Build history of the part. All positions in model axes, mm. A direction names the side the tool comes from. Coordinates: 2 decimals unless noted, no trailing zeros.
```python
from build123d import *

# Parameters (mm, degrees)
SKETCH_W        = 150
SKETCH_H        = 115
PAD_DEPTH       = 3
SKETCH001_W     = 150
SKETCH001_H     = 3
PAD001_DEPTH    = 40
SKETCH002_R     = 3.5
SKETCH002_R_2   = 1.5
PAD002_DEPTH    = 7
SKETCH003_R     = 8.2
SKETCH003_R_2   = 2.25
POCKET_DEPTH    = 5
SKETCH004_R     = 3.65
SKETCH004_R_2   = 1.6
POCKET001_DEPTH = 5
PAD003_DEPTH    = 9
POCKET002_DEPTH = 8
SKETCH007_R     = 2.956815
SKETCH007_R_2   = 3.91912
POCKET003_DEPTH = 5
SKETCH008_R     = 3.375
POCKET004_DEPTH = 5
POCKET005_DEPTH = 5
SKETCH012_W     = 6
SKETCH012_H     = 8
PAD006_DEPTH    = 8
SKETCH013_W     = 6
SKETCH013_H     = 8
PAD007_DEPTH    = 8
SKETCH016_R     = 1.5
POCKET008_DEPTH = 10
SKETCH017_R     = 1.5
POCKET009_DEPTH = 10
FILLET001_R     = 2
FILLET002_R     = 1.5


with BuildPart() as part:
    # Sketch → Pad (new body)
    with BuildSketch(Plane.XY):
        with Locations((99.883204, -84.177484)):
            Rectangle(SKETCH_W, SKETCH_H)
    extrude(amount=PAD_DEPTH)

    # Sketch001 (on Face6 of Pad) → Pad001 (join)
    with BuildSketch(Plane.XY.offset(3)):
        with Locations((99.883211, -140.17749)):
            Rectangle(SKETCH001_W, SKETCH001_H)
        with Locations((99.883211, -28.1775)):
            Rectangle(SKETCH001_W, SKETCH001_H)
    extrude(amount=PAD001_DEPTH)

    # Sketch002 (on Face5 of Pad001) → Pad002 (join)
    with BuildSketch(Plane.XY.offset(3)):
        with Locations((45.316391, -43.665684)):
            Circle(SKETCH002_R)
        with Locations((45.316391, -43.665684)):
            Circle(SKETCH002_R_2, mode=Mode.SUBTRACT)
        with Locations((134.578049, -43.803013)):
            Circle(SKETCH002_R)
        with Locations((134.578049, -43.803013)):
            Circle(SKETCH002_R_2, mode=Mode.SUBTRACT)
        with Locations((45.316391, -133.064651)):
            Circle(SKETCH002_R)
        with Locations((45.316391, -133.064651)):
            Circle(SKETCH002_R_2, mode=Mode.SUBTRACT)
        with Locations((134.578049, -132.927338)):
            Circle(SKETCH002_R)
        with Locations((134.578049, -132.927338)):
            Circle(SKETCH002_R_2, mode=Mode.SUBTRACT)
    extrude(amount=PAD002_DEPTH)

    # Sketch003 (on Face8 of Pad002) → Pocket (cut)
    with BuildSketch(Plane(origin=(0, -26.6775, 0), x_dir=(-1, 0, 0), z_dir=(0, 1, 0))):
        with Locations((-155.160995, 22.957462)):
            Circle(SKETCH003_R)
        with Locations((-128.150894, 23.01816)):
            Circle(SKETCH003_R)
        with Locations((-164.297668, 32.157272)):
            Circle(SKETCH003_R_2)
        with Locations((-145.858627, 32.062714)):
            Circle(SKETCH003_R_2)
        with Locations((-164.113113, 13.90062)):
            Circle(SKETCH003_R_2)
        with Locations((-145.905151, 13.821107)):
            Circle(SKETCH003_R_2)
        with Locations((-137.079453, 32.188087)):
            Circle(SKETCH003_R_2)
        with Locations((-137.091354, 13.88285)):
            Circle(SKETCH003_R_2)
        with Locations((-118.778183, 32.004562)):
            Circle(SKETCH003_R_2)
        with Locations((-118.969612, 14.010464)):
            Circle(SKETCH003_R_2)
        with Locations((-109.972557, 13.819037)):
            Circle(SKETCH003_R_2)
        with Locations((-109.969048, 32.209045)):
            Circle(SKETCH003_R_2)
        with Locations((-91.723251, 32.195992)):
            Circle(SKETCH003_R_2)
        with Locations((-91.787064, 13.88285)):
            Circle(SKETCH003_R_2)
        with Locations((-101.261856, 22.888664)):
            Circle(SKETCH003_R)
    extrude(amount=-POCKET_DEPTH, mode=Mode.SUBTRACT)

    # Sketch004 (on Face19 of Pocket) → Pocket001 (cut)
    with BuildSketch(Plane.XZ.offset(141.67749)):
        with Locations((87.170862, 25.966157)):
            Circle(SKETCH004_R)
        with Locations((124.674583, 25.581327)):
            Circle(SKETCH004_R)
        with Locations((61.41629, 22.568558)):
            Circle(SKETCH004_R_2)
        with Locations((54.032642, 22.454962)):
            Circle(SKETCH004_R_2)
    extrude(amount=-POCKET001_DEPTH, mode=Mode.SUBTRACT)

    # Sketch005 (on Face8 of Pocket001) → Pad003 (join)
    with BuildSketch(Plane(origin=(0, -26.6775, 0), x_dir=(-1, 0, 0), z_dir=(0, 1, 0))):
        with BuildLine():
            ThreePointArc((-71.425017, 25.728505), (-79.425017, 17.728505), (-71.425017, 9.728505))
            Line((-71.425017, 9.728505), (-56.425017, 9.728505))
            ThreePointArc((-56.425017, 9.728505), (-48.425017, 17.728505), (-56.425017, 25.728505))
            Line((-71.425017, 25.728505), (-56.425017, 25.728505))
        make_face()
    extrude(amount=-PAD003_DEPTH)

    # Sketch006 (on Face58 of Pad003) → Pocket002 (cut)
    with BuildSketch(Plane(origin=(0, -26.6775, 0), x_dir=(-1, 0, 0), z_dir=(0, 1, 0))):
        with BuildLine():
            ThreePointArc((-71.144104, 24.608639), (-78.144104, 17.608639), (-71.144104, 10.608639))
            Line((-71.144104, 10.608639), (-56.644104, 10.608639))
            ThreePointArc((-56.644104, 10.608639), (-49.644104, 17.608639), (-56.644104, 24.608639))
            Line((-71.144104, 24.608639), (-56.644104, 24.608639))
        make_face()
    extrude(amount=-POCKET002_DEPTH, mode=Mode.SUBTRACT)

    # Sketch007 (on Face54 of Pocket002) → Pocket003 (cut)
    with BuildSketch(Plane(origin=(0, -34.6775, 0), x_dir=(-1, 0, 0), z_dir=(0, 1, 0))):
        with Locations((-71.614014, 15.088903)):
            Circle(SKETCH007_R)
        with Locations((-56.978443, 19.166483)):
            Circle(SKETCH007_R_2)
    extrude(amount=-POCKET003_DEPTH, mode=Mode.SUBTRACT)

    # Sketch008 (on Face19 of Pocket003) → Pocket004 (cut)
    with BuildSketch(Plane.XZ.offset(141.67749)):
        with Locations((161.787576, 25.778181)):
            Circle(SKETCH008_R)
        with Locations((35.800133, 25.778181)):
            Circle(SKETCH008_R)
        with Locations((105.628538, 25.778181)):
            Circle(SKETCH008_R)
        with Locations((145.6931, 25.778181)):
            Circle(SKETCH008_R)
    extrude(amount=-POCKET004_DEPTH, mode=Mode.SUBTRACT)

    # Sketch009 (on Face5 of Pocket004) → Pocket005 (cut)
    with BuildSketch(Plane.XY.offset(3)):
        with BuildLine():
            ThreePointArc((39.81937, -90.12404), (42.31937, -92.62404), (44.81937, -90.12404))
            Line((44.81937, -90.12404), (44.81937, -60.12404))
            ThreePointArc((44.81937, -60.12404), (42.31937, -57.62404), (39.81937, -60.12404))
            Line((39.81937, -90.12404), (39.81937, -60.12404))
        make_face()
        with BuildLine():
            ThreePointArc((47.81937, -90.124041), (50.31937, -92.624041), (52.81937, -90.124041))
            Line((52.81937, -90.124041), (52.81937, -60.124041))
            ThreePointArc((52.81937, -60.124041), (50.31937, -57.624041), (47.81937, -60.124041))
            Line((47.81937, -90.124041), (47.81937, -60.124041))
        make_face()
        with BuildLine():
            ThreePointArc((55.81937, -90.12404), (58.31937, -92.62404), (60.81937, -90.12404))
            Line((60.81937, -90.12404), (60.81937, -60.12404))
            ThreePointArc((60.81937, -60.12404), (58.31937, -57.62404), (55.81937, -60.12404))
            Line((55.81937, -90.12404), (55.81937, -60.12404))
        make_face()
        with BuildLine():
            ThreePointArc((63.81937, -90.124041), (66.31937, -92.624041), (68.81937, -90.124041))
            Line((68.81937, -90.124041), (68.81937, -60.124041))
            ThreePointArc((68.81937, -60.124041), (66.31937, -57.624041), (63.81937, -60.124041))
            Line((63.81937, -90.124041), (63.81937, -60.124041))
        make_face()
        with BuildLine():
            ThreePointArc((71.81937, -90.12404), (74.31937, -92.62404), (76.81937, -90.12404))
            Line((76.81937, -90.12404), (76.81937, -60.12404))
            ThreePointArc((76.81937, -60.12404), (74.31937, -57.62404), (71.81937, -60.12404))
            Line((71.81937, -90.12404), (71.81937, -60.12404))
        make_face()
        with BuildLine():
            ThreePointArc((79.81937, -90.12404), (82.31937, -92.62404), (84.81937, -90.12404))
            Line((84.81937, -90.12404), (84.81937, -60.12404))
            ThreePointArc((84.81937, -60.12404), (82.31937, -57.62404), (79.81937, -60.12404))
            Line((79.81937, -90.12404), (79.81937, -60.12404))
        make_face()
    extrude(amount=-POCKET005_DEPTH, mode=Mode.SUBTRACT)

    # Sketch012 (on Face35 of Pocket005) → Pad006 (join)
    with BuildSketch(Plane.XZ.offset(29.6775)):
        with Locations((168.598978, 7.25481)):
            Rectangle(SKETCH012_W, SKETCH012_H)
        with Locations((30.984795, 7.198986)):
            Rectangle(SKETCH012_W, SKETCH012_H)
    extrude(amount=PAD006_DEPTH)

    # Sketch013 (on Face36 of Pad006) → Pad007 (join)
    with BuildSketch(Plane(origin=(0, -138.67749, 0), x_dir=(-1, 0, 0), z_dir=(0, 1, 0))):
        with Locations((-30.980019, 7.152398)):
            Rectangle(SKETCH013_W, SKETCH013_H)
        with Locations((-168.610458, 7.248077)):
            Rectangle(SKETCH013_W, SKETCH013_H)
    extrude(amount=PAD007_DEPTH)

    # Sketch016 (on Face73 of Pad007) → Pocket008 (cut)
    with BuildSketch(Plane(origin=(27.984795, 0, 0), x_dir=(0, -1, 0), z_dir=(-1, 0, 0))):
        with Locations((33.567612, 7.141162)):
            Circle(SKETCH016_R)
        with Locations((134.571213, 7.150399)):
            Circle(SKETCH016_R)
    extrude(amount=-POCKET008_DEPTH, mode=Mode.SUBTRACT)

    # Sketch017 (on Face89 of Pocket008) → Pocket009 (cut)
    with BuildSketch(Plane.YZ.offset(171.610458)):
        with Locations((-134.832733, 7.230164)):
            Circle(SKETCH017_R)
        with Locations((-33.852489, 7.223049)):
            Circle(SKETCH017_R)
    extrude(amount=-POCKET009_DEPTH, mode=Mode.SUBTRACT)

    # Fillet001
    fillet001_edges = [part.edges().sort_by_distance(p)[0] for p in [
        (24.883204, -84.177484, 0),
        (24.883211, -28.1775, 43),
        (24.883211, -140.17749, 43),
        (174.883211, -140.17749, 43),
        (174.883204, -84.177484, 0),
        (174.883211, -28.1775, 43),
    ]]
    fillet(fillet001_edges, radius=FILLET001_R)

    # Fillet002
    fillet002_edges = [part.edges().sort_by_distance(p)[0] for p in [
        (63.894104, -26.6775, 24.608639),
        (49.644104, -26.6775, 17.608639),
        (63.894104, -26.6775, 10.608639),
        (78.144104, -26.6775, 17.608639),
    ]]
    fillet(fillet002_edges, radius=FILLET002_R)


solid = part.part
```
1. Saw through at A-A on y = -63. State how many separate pieces and enclosed holes the cut face has, plus the area to 3 significant figures.
Computed values:
separate pieces: 7
enclosed holes: 0
area: 358 mm2
2. Mould opens along Z. For faces 5 (the face through (99, -83, 0)), 6 (the face through (169, -34, 3.255)), 7 (the face through (47.819, -75, 2)) say: +Z half, -Z half, draft (parallel to the pull), parting line (faces both ways), or undercut.
Computed values:
face 5: -Z half
face 6: undercut
face 7: draft
3. 3-axis set-ups, long thin cutter, end or side, ignore diameter. For faces 1 (the face through (58.374, -57.625, 1.521)), 2 (the face through (148.912, -140.198, 26.792)), 3 (the face through (163.353, -28.156, 23.318)), 4 (the face through (47, -133, 10)): which of +Z, -Z, +X, -X, +Y, -Y reach the whole face in a straight line?
Computed values:
face 1: +Z, -Z
face 2: -Y
face 3: +Y
face 4: +Z
4. Flat gauge pins, fed straight in: pin 1 (3.5 mm diameter, centred on x = 54.03, z = 22.45, fed in from +Y); pin 2 (1.8 mm diameter, centred on y = -33.57, z = 7.14, fed in from -X); pin 3 (3.5 mm diameter, centred on x = 134.5, y = -132.5, fed in from +Z); pin 4 (8 mm diameter, centred on x = 94.5, y = -51.5, fed in from +Z). Where does each tip first touch, or does it go through?
Computed values:
pin 1: stops at y = -27.35
pin 2: passes through
pin 3: stops at z = 10
pin 4: stops at z = 3
5. Probe line 1 along Y through (x, z) = (39, 29.5); line 2 along Z through (x, y) = (65, -121); line 3 along Y through (x, z) = (55.5, 10). List the from-to ranges inside material, lowest first.
Computed values:
line 1: y = -141.68 to -138.68, -29.68 to -26.68
line 2: z = 0 to 3
line 3: y = -141.68 to -138.68, -35.68 to -26.91
